from build123d import *

# Parameters (mm, degrees)
SKETCH1_W               = 40
SKETCH1_H               = 20
BOSS_EXTRUDE1_DEPTH     = 35
FILLET1_RADIUS          = 20
FILLET1_LENGTH          = 20
CUT_EXTRUDE1_DEPTH      = 42.533119315
CUT_EXTRUDE1_DEPTH_BACK = 42.533119315
CUT_EXTRUDE2_DEPTH      = 42.533119315
CUT_EXTRUDE2_DEPTH_BACK = 42.533119315
FILLET2_R               = 10
FILLET3_R               = 10
SKETCH7_R               = 0.7
CUT_EXTRUDE3_DEPTH      = 35
SKETCH10_R              = 0.5
CUT_EXTRUDE4_DEPTH      = 5


with BuildPart() as part:
    # Sketch1 → Boss-Extrude1 (new body)
    with BuildSketch(Plane.XY):
        Rectangle(SKETCH1_W, SKETCH1_H)
    extrude(amount=BOSS_EXTRUDE1_DEPTH)

    # Fillet1: full round fillet: the end face becomes a half cylinder, R = half its width
    fillet1_face = Plane((0, 0, 35), x_dir=(0, -1, 0), z_dir=(0, 0, 1))  # on the end face: x along it, z out of the body
    fillet1_slab = fillet1_face.offset(-FILLET1_RADIUS / 2) * Box(FILLET1_LENGTH, 2 * FILLET1_RADIUS, FILLET1_RADIUS, mode=Mode.PRIVATE)  # the body's end, R deep
    fillet1_round = Plane((0, 0, 15), x_dir=(0, 0, 1), z_dir=(0, -1, 0)) * Cylinder(FILLET1_RADIUS, FILLET1_LENGTH, mode=Mode.PRIVATE)  # its axis R under the face
    add(fillet1_slab - fillet1_round, mode=Mode.SUBTRACT)

    # Sketch3 → Cut-Extrude1 (cut, two sides: drawn at the far end of the back side and taken through both)
    with BuildSketch(Plane(origin=(0, 0, 0), x_dir=(1, 0, 0), z_dir=(0, 1, 0)).offset(-CUT_EXTRUDE1_DEPTH_BACK)):
        Polygon((-12.624608069, -34.987358945), (-18.720278541, 4.574737646), (-30.971557894, -1.916976114), (-24.875887422, -41.479072706), align=None)
    extrude(amount=CUT_EXTRUDE1_DEPTH + CUT_EXTRUDE1_DEPTH_BACK, mode=Mode.SUBTRACT)

    # Sketch4 → Cut-Extrude2 (cut, two sides: drawn at the far end of the back side and taken through both)
    with BuildSketch(Plane(origin=(0, 0, 0), x_dir=(1, 0, 0), z_dir=(0, 1, 0)).offset(-CUT_EXTRUDE2_DEPTH_BACK)):
        Polygon((11.956946172, -36.772482669), (19.210484507, 7.59218203), (33.970591583, -6.999238108), (26.717053249, -51.363902807), align=None)
    extrude(amount=CUT_EXTRUDE2_DEPTH + CUT_EXTRUDE2_DEPTH_BACK, mode=Mode.SUBTRACT)

    # Fillet2
    fillet2_edges = [part.edges().sort_by_distance(p)[0] for p in [
        (13.036926478, 0, 30.167021725),
    ]]
    fillet(fillet2_edges, radius=FILLET2_R)

    # Fillet3
    fillet3_edges = [part.edges().sort_by_distance(p)[0] for p in [
        (-13.419277094, 0, 29.829801154),
    ]]
    fillet(fillet3_edges, radius=FILLET3_R)

    # Sketch7 → Cut-Extrude3 (cut)
    with BuildSketch(Plane.XY.offset(33)):
        with Locations(Location((0, 0, 0), (0, 0, 180))):
            Circle(SKETCH7_R)
    extrude(amount=CUT_EXTRUDE3_DEPTH, mode=Mode.SUBTRACT)

    # Sketch10 → Cut-Extrude4 (cut)
    with BuildSketch(Plane.XY):
        with Locations((-5, 0)):
            Circle(SKETCH10_R)
        with Locations(Location((5, 0, 0), (0, 0, 180))):
            Circle(SKETCH10_R)
    extrude(amount=CUT_EXTRUDE4_DEPTH, mode=Mode.SUBTRACT)


solid = part.part
Check sheet for the modelled part. Datum: model origin and axes. Units: mm. A direction names the side the tool comes from. Give positions to 0.01 mm unless a question says otherwise; leave off trailing zeros. Write each loop counter-clockwise with the first axis right and the second up, starting at its lowest first coordinate (ties: lowest second). Pieces come first, ordered by that corner, then holes. Notation, with made-up numbers: M 19,10.5 L 36,10.5 A14 ccw 36,25.5 Z; hole C 45,39.5 d1. An arc over 180 degrees is marked long. Use one line per item in the form item = value.
(1) Draft check along X on faces 4 (the cylindrical face through (-5.4, -0.3, 2.5)), 5 (the cylindrical face through (-12.131, -0.14, 30.155)), 6 (the flat face through (0, 10, 17)). Enter one of: pulls with the +X half, pulls with the -X half, needs draft (parallel to the pull), parting line crosses it, or undercut.
Answer block:
face_4 = undercut
face_5 = pulls with the -X half
face_6 = needs draft
(2) Section check A-A on y = -7.25. Record the boundary of the cut face in (x, z), plus the area to 3 significant figures.
Answer block:
outline = M -18.02,0 L 17.97,0 L 13.75,25.83 A10 ccw 7.75,33.44 A20 ccw -8.37,33.16 A10 ccw -14.07,25.6 Z
area = 1,020 mm2
(3) Section check D-D on y = 0. Record the boundary of the cut face in (x, z), plus the area to 3 significant figures.
Answer block:
outline = M -18.02,0 L -5.5,0 L -5.5,5 L -4.5,5 L -4.5,0 L 4.5,0 L 4.5,5 L 5.5,5 L 5.5,0 L 17.97,0 L 13.75,25.83 A10 ccw 7.75,33.44 A20 ccw 0.7,34.99 L 0.7,33 L -0.7,33 L -0.7,34.99 A20 ccw -8.37,33.16 A10 ccw -14.07,25.6 Z
area = 1,010 mm2
(4) Tool access check on faces 1 (the flat face through (0, -10, 17)), 2 (the flat face through (5, 0, 5)), 3 (the flat face through (0, 0, 33)). Record the directions out of +Z, -Z, +X, -X, +Y, -Y that give a thin tool (end or side, any length) a straight path to the whole face; none if there is none.
Answer block:
face_1 = +Z, -Z, +X, -X, -Y
face_2 = -Z
face_3 = +Z
(5) Depth check by flat-ended pin: P1, Ø5, axis at x = -9, y = 3.5, coming from the +Z side; P2, Ø6, axis at x = -11.5, y = 2.5, coming from the +Z side; P3, Ø4, axis at x = 13, y = -0.5, coming from the +Z side. Enter the tip coordinate at first touch or a pass-through.
Answer block:
P1 = 33.91
P2 = 33.1
P3 = 31.24
(6) Material ranges on line 1 along Y through (x, z) = (0, 33.55); line 2 along Y through (x, z) = (5, 3.35); line 3 along Z through (x, y) = (-8, -7), recorded low to high.
Answer block:
line_1 = -10 to -0.7, 0.7 to 10
line_2 = -10 to -0.5, 0.5 to 10
line_3 = 0 to 33.33
(7) Section check C-C on z = 14.5. Record the boundary of the cut face in (x, y).
Answer block:
outline = M -15.78,-10 L 15.6,-10 L 15.6,10 L -15.78,10 Z
(8) Section check B-B on x = -5. Record the boundary of the cut face in (y, z).
Answer block:
outline = M -10,0 L -0.5,0 L -0.5,5 L 0.5,5 L 0.5,0 L 10,0 L 10,34.36 L -10,34.36 Z
